Autodesk Inventor part; units mm, degrees
ref_plane "YZ Plane" through (0, 0, 0) normal (1, 0, 0) x (0, 1, 0)
ref_plane "XZ Plane" through (0, 0, 0) normal (0, 1, 0) x (-1, 0, 0)
ref_plane "XY Plane" through (0, 0, 0) normal (0, 0, 1) x (1, 0, 0)
sketch "Sketch1" plane through (0, 0, 0) normal (0, 0, 1) x (1, 0, 0)
  arc A0 (-44.218038, -12.679318) -> (-22.234092, -40.269655) centre (0, 0) ccw construction
  arc A1 (-22.234092, -40.269655) -> (-40.195246, 22.368331) centre (-70.172104, -20.121527) ccw
  line L0 (0, 0) -> (-70.172104, -20.121527) construction
  line L1 (0, -64.4) -> (0, 64.4) construction
  arc A2 (40.195246, 22.368331) -> (22.234092, -40.269655) centre (70.172104, -20.121527) ccw
  line L2 (0, 0) -> (70.172104, -20.121527) construction
  arc A3 (-40.195246, 22.368331) -> (-44.218038, 12.679318) centre (0, 0) ccw construction
  arc A4 (-22.234092, -40.269655) -> (22.234092, -40.269655) centre (0, 0) ccw
  arc A5 (22.234092, -40.269655) -> (40.195246, 22.368331) centre (0, 0) ccw construction
  arc A6 (40.195246, 22.368331) -> (-40.195246, 22.368331) centre (0, 0) ccw
  arc A7 (-44.218038, 12.679318) -> (-44.218038, -12.679318) centre (0, 0) ccw construction
  dimension "d0" = 92
  dimension "d1" = 52
  dimension "d2" = 73
  dimension "d3" = 148
extrude "Extrusion1" add sketch "Sketch1" along normal mid plane 10
sketch "Sketch2" plane through (0, 0, 5) normal (0, 0, 1) x (1, 0, 0)
  arc A0 (-22.234092, -40.269655) -> (-40.195246, 22.368331) centre (-70.172104, -20.121527) ccw
  arc A1 (-22.234092, -40.269655) -> (22.234092, -40.269655) centre (0, 0) ccw
  arc A2 (40.195246, 22.368331) -> (22.234092, -40.269655) centre (70.172104, -20.121527) ccw
  arc A3 (40.195246, 22.368331) -> (-40.195246, 22.368331) centre (0, 0) ccw
  line L0 (0, 0) -> (-70.172104, -20.121527) construction
  line L1 (0, 0) -> (70.172104, -20.121527) construction
  point P0 (-14.418925, -4.13456)
  point P1 (14.418925, -4.13456)
  dimension "d6" = 15
  dimension "d7" = 15
hole "Hole1" at (-14.418925, -4.13456, 5) at (14.418925, -4.13456, 5) direction (0, 0, -1) diameter 4 end through all
sketch "Sketch3" plane through (0, 0, 5) normal (0, 0, 1) x (1, 0, 0)
  arc A0 (-22.234092, -40.269655) -> (22.234092, -40.269655) centre (0, 0) ccw
hole "Hole2" at (0, 0, 5) direction (0, 0, -1) diameter 9 end through all
chamfer "Chamfer1" distance 0.5 angle 45 4 edges at (0, 46, 5) (0, 46, -5) (0, -46, -5) (0, -46, 5)
sketch "Sketch4" plane through (0, 0, 5) normal (0, 0, 1) x (1, 0, 0)
  arc A0 (-22.041384, -39.804866) -> (22.041384, -39.804866) centre (0, 0) ccw
  arc A1 (39.785519, 22.076287) -> (22.041384, -39.804866) centre (70.172104, -20.121527) ccw
  arc A2 (39.785519, 22.076287) -> (-39.785519, 22.076287) centre (0, 0) ccw
  arc A3 (-22.041384, -39.804866) -> (-39.785519, 22.076287) centre (-70.172104, -20.121527) ccw
  circle A4 centre (0, 0) radius 4.5
  circle A5 centre (-14.418925, -4.13456) radius 2
  circle A6 centre (14.418925, -4.13456) radius 2
  arc A7 (37.160523, 22.61295) -> (-37.160523, 22.61295) centre (0, 0) ccw
  arc A8 (37.160523, 22.61295) -> (19.530873, -38.868946) centre (70.172104, -20.121527) ccw
  arc A9 (-19.530873, -38.868946) -> (19.530873, -38.868946) centre (0, 0) ccw
  arc A10 (-19.530873, -38.868946) -> (-37.160523, 22.61295) centre (-70.172104, -20.121527) ccw
  circle A11 centre (-14.418925, -4.13456) radius 4
  circle A12 centre (0, 0) radius 6.5
  circle A13 centre (14.418925, -4.13456) radius 4
  dimension "d25" = 2
  dimension "d26" = 2
  dimension "d27" = 2
  dimension "d28" = 2
extrude "Extrusion2" cut sketch "Sketch4" against normal blind 0.5 contours A8 A9 A10 A7
mirror "Mirror1" about plane through (0, 0, 0) normal (0, 0, 1) of "Extrusion2"
properties part number "Disk" material "Steel"
Design review of the part built by this model. Coordinates are the model's own, in mm. A direction names the side the tool comes from. Coordinates: 2 decimals unless noted, no trailing zeros. Write each loop counter-clockwise with the first axis right and the second up, starting at its lowest first coordinate (ties: lowest second). Pieces come first, ordered by that corner, then holes. Notation, with made-up numbers: (-22.75, 48) -> (-10.75, 48) arc R26 cw to (-10.75, 85) -> close; hole circle Ø10 at (72.25, 32.25). An arc over 180 degrees is marked (long way). Write each question's results on one line, items separated by ' | '. Start each with the question number.
(1) Take a section at D-D on y = 15.5. Write out the cut boundary in (x, z).
(2) Take a section at B-B on z = 3. Write out the cut boundary in (x, y).
(3) Take a section at A-A on x = 0. Write out the cut boundary in (y, z), and give its area (4 significant figures).
(4) Clearance check with flat-ended pins moving along their axes: P1, Ø3, axis at x = -23.5, z = -4, coming from the -Y side; P2, Ø6, axis at x = 11.5, z = 4, coming from the +Y side; P3, Ø2.5, axis at x = 14.42, y = -4.13, coming from the +Z side; P4, Ø3, axis at x = -21.5, y = 32, coming from the +Z side. State where each tip first meets the part, or that it passes through.
(5) Tool access review of faces 5 (the face through (15, -2, -5)), 6 (the face through (-0.3, -43.5, 4.8)), 7 (the face through (-5.158, 3.955, -4.754)): name each direction out of +Z, -Z, +X, -X, +Y, -Y from which nothing blocks a thin tool from reaching the whole face with its end or side.
(6) For line 1 along Z through (x, y) = (-21, 30.5); line 2 along Y through (x, z) = (0, -0.5); line 3 along Y through (x, z) = (14, 2.5), list the stretches that pass through material, from the lowest coordinate up. Write a range as from..to.
(7) The part is to be moulded in two halves that separate along X. For faces 1 (the face through (-14, -2, -5)), 2 (the face through (-0.68, 45.637, 4.858)), 3 (the face through (-4.46, 0.59, -0.07)), 4 (the face through (-0.624, 43.496, -4.754)), say which applies: pulls with the +X half, pulls with the -X half, needs draft (parallel to the pull), parting line crosses it, or undercut.
(8) Take a section at C-C on y = -12.5. Write out the cut boundary in (x, z).
Results found:
1) outline: (-32.29, -5) -> (-29.59, -5) -> (-29.59, -4.5) -> (29.59, -4.5) -> (29.59, -5) -> (32.29, -5) -> (32.29, 5) -> (29.59, 5) -> (29.59, 4.5) -> (-29.59, 4.5) -> (-29.59, 5) -> (-32.29, 5) -> close
2) outline: (-40.2, 22.37) arc R52 cw to (-22.23, -40.27) arc R46 ccw to (22.23, -40.27) arc R52 cw to (40.2, 22.37) arc R46 ccw to start; hole circle Ø4 at (-14.42, -4.13); hole circle Ø9 at (0, 0); hole circle Ø4 at (14.42, -4.13)
3) outline: (-46, -4.5) -> (-45.5, -5) -> (-43.5, -5) -> (-43.5, -4.5) -> (-6.5, -4.5) -> (-6.5, -5) -> (-4.5, -5) -> (-4.5, 5) -> (-6.5, 5) -> (-6.5, 4.5) -> (-43.5, 4.5) -> (-43.5, 5) -> (-45.5, 5) -> (-46, 4.5) -> close; (4.5, -5) -> (6.5, -5) -> (6.5, -4.5) -> (43.5, -4.5) -> (43.5, -5) -> (45.5, -5) -> (46, -4.5) -> (46, 4.5) -> (45.5, 5) -> (43.5, 5) -> (43.5, 4.5) -> (6.5, 4.5) -> (6.5, 5) -> (4.5, 5) -> close | area: 755.5 mm2
4) P1: stops at y = -40.4 | P2: stops at y = 45.21 | P3: passes through | P4: stops at z = 4.5
5) face 5: -Z, +X, -X, +Y, -Y | face 6: +Z | face 7: -Z
6) line 1: z = -4.5..4.5 | line 2: y = -46..-4.5, 4.5..46 | line 3: y = -43.82..-6.09, -2.18..43.82
7) face 1: needs draft | face 2: parting line crosses it | face 3: undercut | face 4: undercut
8) outline: (-18.73, -5) -> (-16.71, -5) -> (-16.71, -4.5) -> (16.71, -4.5) -> (16.71, -5) -> (18.73, -5) -> (18.73, 5) -> (16.71, 5) -> (16.71, 4.5) -> (-16.71, 4.5) -> (-16.71, 5) -> (-18.73, 5) -> close
